```python
from build123d import *

# Parameters (mm, degrees)
SKETCH1_W           = 40.35
SKETCH1_H           = 43.35
BOSS_EXTRUDE1_DEPTH = 47
CUT_EXTRUDE2_DEPTH  = 102
FILLET1_R           = 10
CUT_EXTRUDE3_DEPTH  = 102
FILLET2_R           = 5
CUT_EXTRUDE5_DEPTH  = 102
SKETCH8_R           = 1.55
CUT_EXTRUDE6_DEPTH  = 102
SKETCH6_R           = 1.5
CUT_EXTRUDE7_DEPTH  = 82.840160626


with BuildPart() as part:
    # Sketch1 → Boss-Extrude1 (new body)
    with BuildSketch(Plane(origin=(0, 0, 0), x_dir=(1, 0, 0), z_dir=(0, 1, 0))):
        with Locations((-26.966212793, -29.108023223)):
            Rectangle(SKETCH1_W, SKETCH1_H)
    extrude(amount=BOSS_EXTRUDE1_DEPTH)

    # Sketch3 → Cut-Extrude2 (cut)
    with BuildSketch(Plane.XY.offset(50.783023223)):
        with BuildLine():
            Line((-47.141212793, 47), (-47.141212793, 26.825))
            ThreePointArc((-47.141212793, 26.825), (-41.232092103, 41.09087931), (-26.966212793, 47))
            Line((-26.966212793, 47), (-47.141212793, 47))
        make_face()
        with BuildLine():
            Line((-6.791212793, 47), (-26.966212793, 47))
            ThreePointArc((-26.966212793, 47), (-12.700333482, 41.09087931), (-6.791212793, 26.825))
            Line((-6.791212793, 26.825), (-6.791212793, 47))
        make_face()
    extrude(amount=-CUT_EXTRUDE2_DEPTH, mode=Mode.SUBTRACT)

    # Fillet1
    fillet1_edges = [part.edges().sort_by_distance(p)[0] for p in [
        (-26.966212793, 0, 50.783023223),
    ]]
    fillet(fillet1_edges, radius=FILLET1_R)

    # Sketch5 → Cut-Extrude3 (cut)
    with BuildSketch(Plane.ZY.offset(47.141212793)):
        with BuildLine():
            Line((-6.665763497, 3.45), (36.595559978, 3.45))
            Line((36.595559978, 3.45), (40.783023223, 3.45))
            ThreePointArc((40.783023223, 3.45), (45.41457264, 5.368450583), (47.333023223, 10))
            Line((47.333023223, 10), (47.333023223, 17.578484004))
            Line((47.333023223, 17.578484004), (47.333023223, 59.778436909))
            Line((47.333023223, 59.778436909), (-6.665763497, 59.778436909))
            Line((-6.665763497, 59.778436909), (-6.665763497, 3.45))
        make_face()
    extrude(amount=-CUT_EXTRUDE3_DEPTH, mode=Mode.SUBTRACT)

    # Fillet2
    fillet2_edges = [part.edges().sort_by_distance(p)[0] for p in [
        (-6.791212793, 1.725, 7.433023223),
        (-47.141212793, 1.725, 7.433023223),
    ]]
    fillet(fillet2_edges, radius=FILLET2_R)

    # Sketch7 → Cut-Extrude5 (cut)
    with BuildSketch(Plane.XY.offset(50.783023223)):
        with BuildLine():
            Line((-33.541212793, 33.925), (-33.541212793, 19.945))
            ThreePointArc((-33.541212793, 19.945), (-26.966212793, 13.37), (-20.391212793, 19.945))
            Line((-20.391212793, 19.945), (-20.391212793, 33.925))
            ThreePointArc((-20.391212793, 33.925), (-26.966212793, 40.5), (-33.541212793, 33.925))
        make_face()
    extrude(amount=-CUT_EXTRUDE5_DEPTH, mode=Mode.SUBTRACT)

    # Sketch8 → Cut-Extrude6 (cut)
    with BuildSketch(Plane.XY.offset(50.783023223)):
        with Locations((-34.766212793, 13.372769702)):
            Circle(SKETCH8_R)
        with Locations((-19.166212793, 13.372769702)):
            Circle(SKETCH8_R)
        with BuildLine():
            ThreePointArc((-12.966212793, 26.825), (-11.416212793, 25.275), (-9.866212793, 26.825))
            Line((-9.866212793, 26.825), (-12.966212793, 26.825))
        make_face()
        with BuildLine():
            Line((-12.966212793, 26.825), (-9.866212793, 26.825))
            ThreePointArc((-9.866212793, 26.825), (-11.416212793, 28.375), (-12.966212793, 26.825))
        make_face()
        with BuildLine():
            ThreePointArc((-44.066212793, 26.825), (-42.516212793, 25.275), (-40.966212793, 26.825))
            Line((-40.966212793, 26.825), (-44.066212793, 26.825))
        make_face()
        with BuildLine():
            Line((-44.066212793, 26.825), (-40.966212793, 26.825))
            ThreePointArc((-40.966212793, 26.825), (-42.516212793, 28.375), (-44.066212793, 26.825))
        make_face()
        with Locations((-34.766212793, 40.277230298)):
            Circle(SKETCH8_R)
        with Locations((-19.166212793, 40.277230298)):
            Circle(SKETCH8_R)
    extrude(amount=-CUT_EXTRUDE6_DEPTH, mode=Mode.SUBTRACT)

    # Sketch6 → Cut-Extrude7 (cut, through all)
    with BuildSketch(Plane(origin=(0, 3.45, 0), x_dir=(1, 0, 0), z_dir=(0, 1, 0))):
        with Locations(Location((-41.966212793, -15.433023223, 0), (0, 0, 270))):
            Circle(SKETCH6_R)
        with Locations(Location((-11.966212793, -15.433023223, 0), (0, 0, 270))):
            Circle(SKETCH6_R)
        with Locations(Location((-41.966212793, -39.433023223, 0), (0, 0, 244.158067237))):
            Circle(SKETCH6_R)
        with Locations(Location((-11.966212793, -39.433023223, 0), (0, 0, 295.841932763))):
            Circle(SKETCH6_R)
    extrude(amount=-CUT_EXTRUDE7_DEPTH, mode=Mode.SUBTRACT)


solid = part.part
```
For this review, take the finished solid that the model builds, in its own axes (mm). A direction names the side the tool comes from. Round coordinates to 2 decimals unless told otherwise and drop trailing zeros. Write each loop counter-clockwise with the first axis right and the second up, starting at its lowest first coordinate (ties: lowest second). Pieces come first, ordered by that corner, then holes. Notation, with made-up numbers: (-18, 24) - (11, 24) arc R15 cw to (11, 53) - close; hole circle Ø3 at (88.25, 30.5). An arc over 180 degrees is marked (long way). Answer as CSV lines item,"result". Start each with the question number.
(1) Machinability: for faces 1 (the flat face through (-18, 28, 47.333)), 2 (the cylindrical face through (-26.82, 40.5, 49.08)), 3 (the flat face through (-6.791, 3, 37)), which of the approach directions +Z, -Z, +X, -X, +Y, -Y give a long, thin tool a straight path to every point of the face, cutting with its end or side? Answer none if there is none.
(2) For pin 1 (2.5 mm diameter, centred on x = -19.17, y = 40.28, fed in from -Z); pin 2 (1 mm diameter, centred on x = -38.5, y = 28, fed in from -Z); pin 3 (1.7 mm diameter, centred on y = 30, z = 49.5, fed in from +X); pin 4 (10 mm diameter, centred on x = -28.5, z = 23, fed in from +Y), all flat-tipped, find the tip position at first contact; note any pin that passes through.
(3) Add section A-A, the plane y = 30.5. State the section outline as (x, z) points, plus the area to 3 significant figures.
(4) Add section C-C, the plane y = 39.5. State the section outline as (x, z) points.
(5) Add section D-D, the plane z = 15. State the section outline as (x, y) points, plus the area to 3 significant figures.
(6) For line 1 (X direction, y = 25.5, z = 48.5); line 2 (Y direction, x = -26, z = 24.5); line 3 (Z direction, x = -17, y = 26.5), list the stretches that pass through material, from the lowest coordinate up.
(7) Mouldability with a two-part tool opening along Y and no side actions: class faces 4 (the cylindrical face through (-17.69, 13.84, 49.08)), 5 (the flat face through (-27, 0, 24)), 6 (the flat face through (-47.141, 3, 37)) as +Y half, -Y half, draft (parallel to the pull), parting line (faces both ways), or undercut.
(8) Add section B-B, the plane x = -25. State the section outline as (y, z) points, plus the area to 3 significant figures.
From the geometry:
1,face 1,"-Z, +X, -X, +Y"
1,face 2,"+Z, -Z"
1,face 3,"+Z, -Z, +X, +Y, -Y"
2,pin 1,"passes through"
2,pin 2,"stops at z = 47.33"
2,pin 3,"stops at x = -6.93"
2,pin 4,"stops at y = 3.45"
3,outline,"(-46.8, 47.33) - (-33.54, 47.33) - (-33.54, 50.78) - (-46.8, 50.78) - close; (-20.39, 47.33) - (-7.13, 47.33) - (-7.13, 50.78) - (-20.39, 50.78) - close"
3,area,"91.5 mm²"
4,outline,"(-42.66, 47.33) - (-36.11, 47.33) - (-36.11, 50.78) - (-42.66, 50.78) - close; (-33.43, 47.33) - (-30.45, 47.33) - (-30.45, 50.78) - (-33.43, 50.78) - close; (-23.48, 47.33) - (-20.51, 47.33) - (-20.51, 50.78) - (-23.48, 50.78) - close; (-17.83, 47.33) - (-11.27, 47.33) - (-11.27, 50.78) - (-17.83, 50.78) - close"
5,outline,"(-47.14, 0) - (-43.4, 0) - (-43.4, 3.45) - (-47.14, 3.45) - close; (-40.53, 0) - (-13.4, 0) - (-13.4, 3.45) - (-40.53, 3.45) - close; (-10.53, 0) - (-6.79, 0) - (-6.79, 3.45) - (-10.53, 3.45) - close"
5,area,"119 mm²"
6,line 1,"x = -47.14 to -43.32, -41.71 to -33.54, -20.39 to -12.22, -10.61 to -6.79"
6,line 2,"y = 0 to 3.45"
6,line 3,"z = 47.33 to 50.78"
7,face 4,"undercut"
7,face 5,"-Y half"
7,face 6,"draft"
8,outline,"(0, 7.43) - (3.45, 7.43) - (3.45, 40.78) arc R6.55 cw to (10, 47.33) - (13.67, 47.33) - (13.67, 50.78) - (10, 50.78) arc R10 ccw to (0, 40.78) - close; (40.2, 47.33) - (46.9, 47.33) - (46.9, 50.78) - (40.2, 50.78) - close"
8,area,"196 mm²"
